The listing builds one solid part. Answer for the finished solid, in the listing's coordinates (mm). A direction names the side the tool comes from. Coordinates: 2 decimals unless noted, no trailing zeros. Order: outer loops, then holes, each group sorted by start corner. A loop starts at its lowest first (then second) coordinate and runs counter-clockwise, first axis right, second up. Notation, with made-up numbers: (-36.5, 25) - (-21.5, 25) arc R22 cw to (-21.5, 34) - close; hole circle Ø9 at (-40, 38.5). An arc over 180 degrees is marked (long way). One line per item, written item: value. Start each with the question number.
```python
from build123d import *

# Parameters (mm, degrees)
EXTRUDE_1_DEPTH     = 14
CUT_EXTRUDE_1_DEPTH = 44
SKETCH_3_W          = 6.2
SKETCH_3_H          = 6.2
CUT_EXTRUDE_2_DEPTH = 4
SKETCH_4_R          = 4
CUT_EXTRUDE_3_DEPTH = 5
SKETCH_5_R          = 2.6
CUT_EXTRUDE_4_DEPTH = 5
SKETCH_6_R          = 4
EXTRUDE_2_DEPTH     = 10
SKETCH_7_W          = 6.2
SKETCH_7_H          = 4
EXTRUDE_3_DEPTH     = 40
CUT_EXTRUDE_5_DEPTH = 50
SKETCH_9_W          = 20
SKETCH_9_H          = 25
EXTRUDE_4_DEPTH     = 44
CUT_EXTRUDE_6_DEPTH = 44
EXTRUDE_5_DEPTH     = 44
SKETCH_12_W         = 6.9
SKETCH_12_H         = 22.5
CUT_EXTRUDE_7_DEPTH = 50
EXTRUDE_START       = 6
EXTRUDE_6_DEPTH     = 6
SKETCH_15_R         = 1.55
CUT_EXTRUDE_8_DEPTH = 2000


with BuildPart() as part:
    # 草图1 → 凸台-拉伸1 (new body)
    with BuildSketch(Plane.XY):
        Polygon((-15, 22), (-15, -22), (15, -22), (15, 22), (0, 22), align=None)
    extrude(amount=EXTRUDE_1_DEPTH)

    # 草图2 → 切除-拉伸1 (cut)
    with BuildSketch(Plane(origin=(0, 22, 0), x_dir=(1, 0, 0), z_dir=(0, 1, 0))):
        Polygon((-15, 0), (-15, -14), (-10, -4), (-3.1, -4), (-3.1, 0), align=None)
        Polygon((3.1, -4), (10, -4), (15, -14), (15, 0), (3.1, 0), align=None)
    extrude(amount=-CUT_EXTRUDE_1_DEPTH, mode=Mode.SUBTRACT)

    # 草图3 → 切除-拉伸2 (cut)
    with BuildSketch(Plane(origin=(0, 0, 0), x_dir=(-1, 0, 0), z_dir=(0, 0, -1))):
        Rectangle(SKETCH_3_W, SKETCH_3_H)
    extrude(amount=-CUT_EXTRUDE_2_DEPTH, mode=Mode.SUBTRACT)

    # 草图4 → 切除-拉伸3 (cut)
    with BuildSketch(Plane.XY.offset(14)):
        Circle(SKETCH_4_R)
    extrude(amount=-CUT_EXTRUDE_3_DEPTH, mode=Mode.SUBTRACT)

    # 草图5 → 切除-拉伸4 (cut)
    with BuildSketch(Plane.XY.offset(9)):
        Circle(SKETCH_5_R)
    extrude(amount=-CUT_EXTRUDE_4_DEPTH, mode=Mode.SUBTRACT)

    # 草图6 → 凸台-拉伸2 (add)
    with BuildSketch(Plane.XY.offset(14)):
        Circle(SKETCH_6_R)
    extrude(amount=-EXTRUDE_2_DEPTH)

    # 草图7 → 凸台-拉伸3 (add)
    with BuildSketch(Plane(origin=(0, -22, 0), x_dir=(-1, 0, 0), z_dir=(0, -1, 0))):
        with Locations((0, -2)):
            Rectangle(SKETCH_7_W, SKETCH_7_H)
    extrude(amount=-EXTRUDE_3_DEPTH)

    # 草图8 → 切除-拉伸5 (cut)
    with BuildSketch(Plane.XZ.offset(22)):
        Polygon((-15, 14), (-10, 4), (-10, 14), align=None)
        Polygon((15, 14), (10, 14), (10, 4), align=None)
    extrude(amount=-CUT_EXTRUDE_5_DEPTH, mode=Mode.SUBTRACT)

    # 草图9 → 凸台-拉伸4 (add)
    with BuildSketch(Plane.XZ.offset(22)):
        with Locations((0, 16.5)):
            Rectangle(SKETCH_9_W, SKETCH_9_H)
    extrude(amount=-EXTRUDE_4_DEPTH)

    # 草图10 → 切除-拉伸6 (cut)
    with BuildSketch(Plane.XZ.offset(22)):
        with BuildLine():
            Line((-10, 29), (-10, 19))
            ThreePointArc((-10, 19), (-7.071067812, 26.071067812), (0, 29))
            Line((0, 29), (-10, 29))
        make_face()
    extrude(amount=-CUT_EXTRUDE_6_DEPTH, mode=Mode.SUBTRACT)

    # 草图11 → 凸台-拉伸5 (add)
    with BuildSketch(Plane.XZ.offset(22)):
        with BuildLine():
            Line((120, 0), (123.1, 0))
            Line((123.1, 0), (123.1, 4))
            Line((123.1, 4), (130, 4))
            Line((130, 4), (130, 19))
            ThreePointArc((130, 19), (127.071067812, 26.071067812), (120, 29))
            Line((120, 29), (110, 29))
            Line((110, 29), (10, 29))
            Line((10, 29), (10, 26.5))
            Line((10, 26.5), (110, 26.5))
            Line((110, 26.5), (110, 4))
            Line((110, 4), (116.9, 4))
            Line((116.9, 4), (116.9, 0))
            Line((116.9, 0), (120, 0))
        make_face()
    extrude(amount=-EXTRUDE_5_DEPTH)

    # 草图12 → 切除-拉伸7 (cut)
    with BuildSketch(Plane(origin=(0, 22, 0), x_dir=(1, 0, 0), z_dir=(0, 1, 0))):
        with Locations((6.55, -15.25)):
            Rectangle(SKETCH_12_W, SKETCH_12_H)
        with Locations((113.45, -15.25)):
            Rectangle(SKETCH_12_W, SKETCH_12_H)
    extrude(amount=-CUT_EXTRUDE_7_DEPTH, mode=Mode.SUBTRACT)

    # 草图14 → 凸台-拉伸6 (add)
    with BuildSketch(Plane(origin=(0, -22, 0), x_dir=(-1, 0, 0), z_dir=(0, -1, 0)).offset(EXTRUDE_START)):
        with BuildLine():
            Line((3.1, 0), (3.1, -4))
            Line((3.1, -4), (10, -4))
            Line((10, -4), (10, -19))
            ThreePointArc((10, -19), (7.071067812, -26.071067812), (0, -29))
            Line((0, -29), (-120, -29))
            ThreePointArc((-120, -29), (-127.071067812, -26.071067812), (-130, -19))
            Line((-130, -19), (-130, -4))
            Line((-130, -4), (-123.1, -4))
            Line((-123.1, -4), (-123.1, 0))
            Line((-123.1, 0), (-116.9, 0))
            Line((-116.9, 0), (-116.9, -26.5))
            Line((-116.9, -26.5), (-3.1, -26.5))
            Line((-3.1, -26.5), (-3.1, 0))
            Line((-3.1, 0), (3.1, 0))
        make_face()
    extrude(amount=-EXTRUDE_6_DEPTH)

    # 草图15 → 切除-拉伸8 (cut)
    with BuildSketch(Plane.ZY.offset(10)):
        with Locations(Location((11.5, 17, 0), (0, 0, 270))):
            Circle(SKETCH_15_R)
        with Locations(Location((11.5, -23, 0), (0, 0, 270))):
            Circle(SKETCH_15_R)
    extrude(amount=-CUT_EXTRUDE_8_DEPTH, mode=Mode.SUBTRACT)


solid = part.part
```
(1) For a pull along Y with two mould halves and no side action, classify faces 5 (the face through (49, 22, 27)), 6 (the face through (61, -3, 26.5)), 7 (the face through (-3.542, -24.432, 10.906)) as pulls with the +Y half, pulls with the -Y half, needs draft (parallel to the pull), parting line crosses it, or undercut.
(2) The part is cut by section C-C on z = 11.5. Determine the outline of the cut face in (x, y), plus the area to 3 significant figures.
(3) Flat-ended cylindrical pins translate along their axes: pin 1 Ø1.5 at (x, y) = (63, -22) entering from -Z; pin 2 Ø3.5 at (x, y) = (128, -2.5) entering from -Z; pin 3 Ø2 at (y, z) = (-6, 2.5) entering from +X; pin 4 Ø2 at (y, z) = (-12.5, 19.5) entering from +X. Find the tip coordinate at first contact, or state that the pin passes through.
(4) For faces 1 (the face through (-3.1, -3, 2)), 2 (the face through (123.1, -3, 2)), 3 (the face through (3.1, -3, 13)), 4 (the face through (130, -3, 12)), determine the directions among +Z, -Z, +X, -X, +Y, -Y from which every point of the face is accessible in a straight line to the end or side of a thin tool.
(5) The part is cut by section D-D on y = 0. Determine the outline of the cut face in (x, z).
(6) Consider probe 1 along X at (y, z) = (-16.5, 13.5); probe 2 along Z at (x, y) = (72.5, 18); probe 3 along Z at (x, y) = (121.75, 17). Determine where each line is inside the solid, lowest interval first.
(7) The part is cut by section B-B on z = 5.5. Determine the outline of the cut face in (x, y), plus the area to 3 significant figures.
(8) The part is cut by section A-A on y = 17. Determine the outline of the cut face in (x, z).
Completed:
1. face 5: pulls with the +Y half
1. face 6: needs draft
1. face 7: undercut
2. outline: (-10, -28) - (3.1, -28) - (3.1, -24.55) - (-10, -24.55) - close; (-10, -21.45) - (3.1, -21.45) - (3.1, 15.45) - (-10, 15.45) - close; (-10, 18.55) - (3.1, 18.55) - (3.1, 22) - (-10, 22) - close; (116.9, -28) - (130, -28) - (130, -24.55) - (116.9, -24.55) - close; (116.9, -21.45) - (130, -21.45) - (130, 15.45) - (116.9, 15.45) - close; (116.9, 18.55) - (130, 18.55) - (130, 22) - (116.9, 22) - close
2. area: 1,150 mm2
3. pin 1: stops at z = 26.5
3. pin 2: stops at z = 4
3. pin 3: stops at x = 123.1
3. pin 4: stops at x = 130
4. face 1: -Z, -X, +Y, -Y
4. face 2: -Z, +X, +Y, -Y
4. face 3: -Z, +Y, -Y
4. face 4: +Z, -Z, +X, +Y, -Y
5. outline: (-10, 4) - (-3.1, 4) - (-3.1, 0) - (3.1, 0) - (3.1, 26.5) - (116.9, 26.5) - (116.9, 0) - (123.1, 0) - (123.1, 4) - (130, 4) - (130, 19) arc R10 ccw to (120, 29) - (0, 29) arc R10 ccw to (-10, 19) - close
6. probe 1: x = -10 to 3.1, 116.9 to 130
6. probe 2: z = 26.5 to 29
6. probe 3: z = 0 to 9.95, 13.05 to 28.85
7. outline: (-10, -28) - (3.1, -28) - (3.1, 22) - (-10, 22) - close; (116.9, -28) - (130, -28) - (130, 22) - (116.9, 22) - close
7. area: 1,310 mm2
8. outline: (-10, 4) - (-3.1, 4) - (-3.1, 0) - (3.1, 0) - (3.1, 9.95) - (-10, 9.95) - close; (-10, 13.05) - (3.1, 13.05) - (3.1, 26.5) - (116.9, 26.5) - (116.9, 13.05) - (130, 13.05) - (130, 19) arc R10 ccw to (120, 29) - (0, 29) arc R10 ccw to (-10, 19) - close; (116.9, 0) - (123.1, 0) - (123.1, 4) - (130, 4) - (130, 9.95) - (116.9, 9.95) - close
